Geometry: see drawing. Coordinates: mm, zero at the bounding-box minimum. Round coordinates to 2 decimals unless told otherwise and drop trailing zeros. Order: outer loops, then holes, each group sorted by start corner. A loop starts at its lowest first (then second) coordinate and runs counter-clockwise, first axis right, second up. Notation, with made-up numbers: (-7.75, 27.5) -> (46.25, 27.5) arc R16 cw to (46.25, 53.5) -> close; hole circle Ø5 at (-29.75, -12). An arc over 180 degrees is marked (long way). One line per item, written item: value. Start each with the question number.
1) Section B-B (x = 4). Return the cut outline in (y, z), and give its area (3 significant figures).
2) Pin query (flat end, axial travel): P1, Ø3, axis at x = 14, z = 1.5, coming from the -Y side; P2, Ø1.5, axis at x = 27.5, y = 19, coming from the +Z side; P3, Ø12, axis at x = 7.5, y = 32, coming from the +Z side. Return the tip coordinate at first contact, or that it passes through.
3) Mould query, pull axis X, two halves, no side actions, for the marked faces 1 and 2. Classes: pulls with the +X half, pulls with the -X half, needs draft (parallel to the pull), parting line crosses it, or undercut.
4) Section A-A (z = 2.5). State how many separate pieces and enclosed holes the cut face has, and give its area (3 significant figures).
5) Ray query, L1, parallel to Y at x = 4, z = 1.6; L2, parallel to X at y = 22.5, z = 0.5; L3, parallel to Y at x = 15, z = 1.5. Return the intervals inside material, ascending.
6) Section D-D (x = 7.9). Return the cut outline in (y, z) (3 decimals).
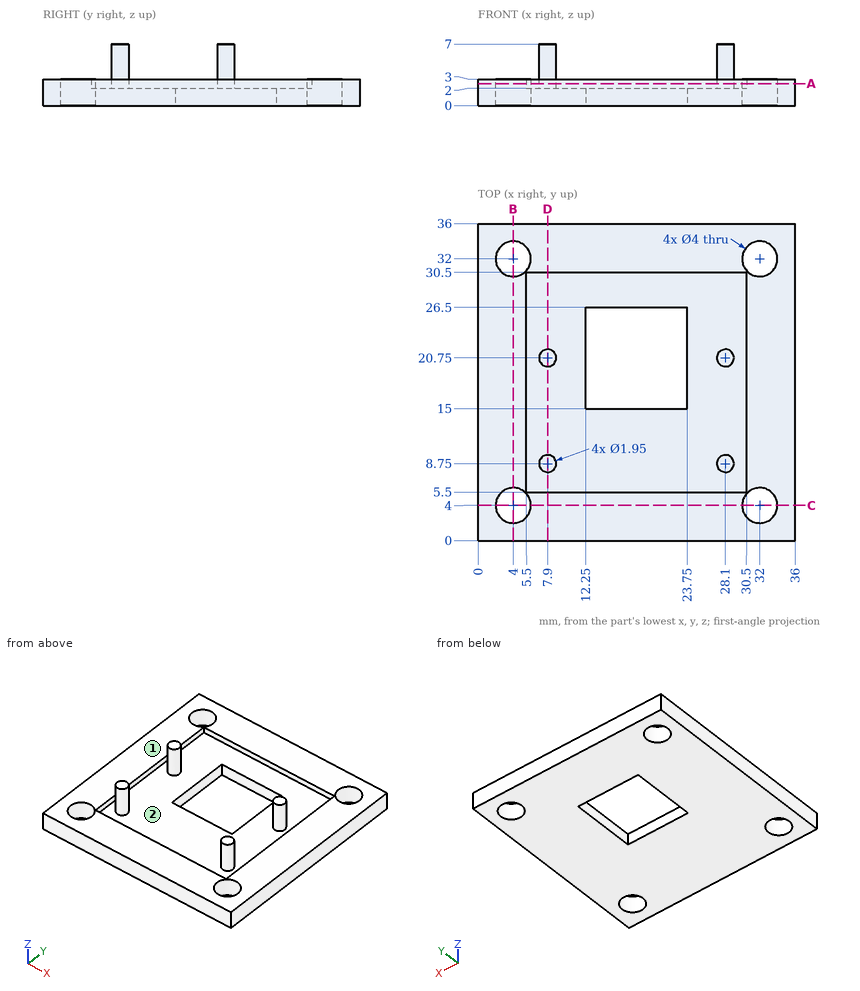
Findings:
1. outline: (0, 0) -> (2, 0) -> (2, 3) -> (0, 3) -> close; (6, 0) -> (30, 0) -> (30, 3) -> (6, 3) -> close; (34, 0) -> (36, 0) -> (36, 3) -> (34, 3) -> close
1. area: 84.0 mm2
2. P1: y = 0
2. P2: z = 2
2. P3: z = 3
3. face 1: needs draft
3. face 2: undercut
4. separate pieces: 5
4. enclosed holes: 5
4. area: 633 mm2
5. L1: 0 to 2, 6 to 30, 34 to 36
5. L2: 0 to 12.25, 23.75 to 36
5. L3: 0 to 15, 26.5 to 36
6. outline: (0, 0) -> (36, 0) -> (36, 3) -> (30.5, 3) -> (30.5, 2) -> (21.725, 2) -> (21.725, 7) -> (19.775, 7) -> (19.775, 2) -> (9.725, 2) -> (9.725, 7) -> (7.775, 7) -> (7.775, 2) -> (5.5, 2) -> (5.5, 3) -> (0, 3) -> close
